Geometry check sheet. Reference: drawing and pictorial views, mm from the part's lowest x, y, z. Round coordinates to 2 decimals unless told otherwise and drop trailing zeros. Order: outer loops, then holes, each group sorted by start corner. A loop starts at its lowest first (then second) coordinate and runs counter-clockwise, first axis right, second up.
Q1. Scan lines: probe 1 along Y at (x, z) = (15, 8); probe 2 along Y at (x, z) = (28.25, 23); probe 3 along Y at (x, z) = (17, 20.25). Record each from-to range of solid material in increasing order.
Q2. Depth check by flat-ended pin: P1, Ø4, axis at x = 3.5, y = 32.5, coming from the +Z side; P2, Ø3, axis at x = 3.69, y = 9.69, coming from the +Z side; P3, Ø1.1, axis at y = 4, z = 24, coming from the +X side; P4, Ø3, axis at x = 6, z = 12.5, coming from the +Y side. Enter the tip coordinate at first touch or a pass-through.
Q3. Cross-section at B-B on x = 30.5. Record the cut outline in (y, z), then the cut area to 3 significant figures.
Q4. Cross-section at D-D on x = 25. Record the cut outline in (y, z), then the cut area to 3 significant figures.
Q5. Cross-section at A-A on y = 21. Record the cut outline in (x, z), then the cut area to 3 significant figures.
Q6. Mould release check, pull along X, two halves, no side actions. Record for the marked faces 1, 2 and 3: +X half, -X half, draft (parallel to the pull), parting line (faces both ways), or undercut.
Q7. Cross-section at C-C on z = 13. Record the cut outline in (x, y), then the cut area to 3 significant figures.
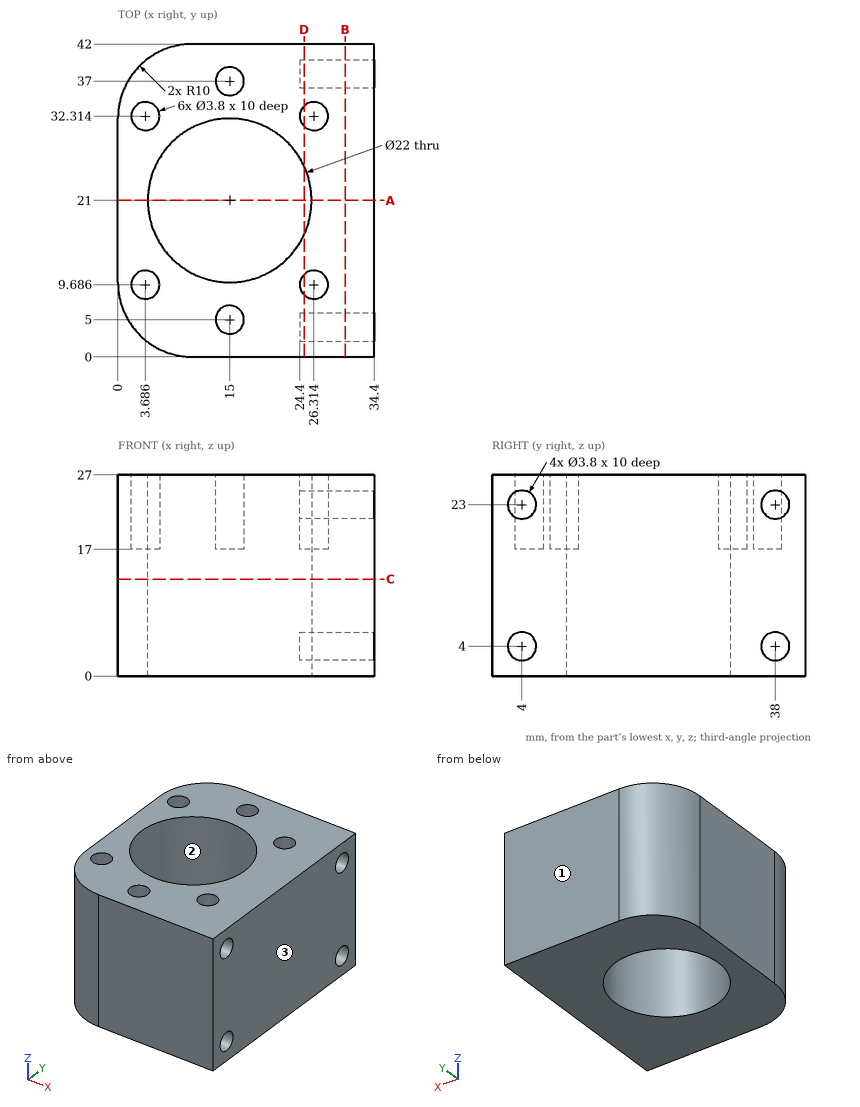
Results found:
1. probe 1: y = 0 to 10, 32 to 42
1. probe 2: y = 0 to 2.1, 5.9 to 36.1, 39.9 to 42
1. probe 3: y = 0 to 10.18, 31.82 to 42
2. P1: stops at z = 27
2. P2: stops at z = 17
2. P3: stops at x = 24.4
2. P4: stops at y = 41.68
3. outline: (0, 0) - (42, 0) - (42, 27) - (0, 27) - close; hole circle Ø3.8 at (4, 4); hole circle Ø3.8 at (4, 23); hole circle Ø3.8 at (38, 4); hole circle Ø3.8 at (38, 23)
3. area: 1,090 mm2
4. outline: (0, 0) - (16.42, 0) - (16.42, 27) - (11.06, 27) - (11.06, 17) - (8.31, 17) - (8.31, 27) - (0, 27) - close; (25.58, 0) - (42, 0) - (42, 27) - (33.69, 27) - (33.69, 17) - (30.94, 17) - (30.94, 27) - (25.58, 27) - close; hole circle Ø3.8 at (4, 4); hole circle Ø3.8 at (4, 23); hole circle Ø3.8 at (38, 4); hole circle Ø3.8 at (38, 23)
4. area: 786 mm2
5. outline: (0, 0) - (4, 0) - (4, 27) - (0, 27) - close; (26, 0) - (34.4, 0) - (34.4, 27) - (26, 27) - close
5. area: 335 mm2
6. face 1: draft
6. face 2: undercut
6. face 3: +X half
7. outline: (0, 10) arc R10 ccw to (10, 0) - (34.4, 0) - (34.4, 42) - (10, 42) arc R10 ccw to (0, 32) - close; hole circle Ø22 at (15, 21)
7. area: 1,020 mm2
